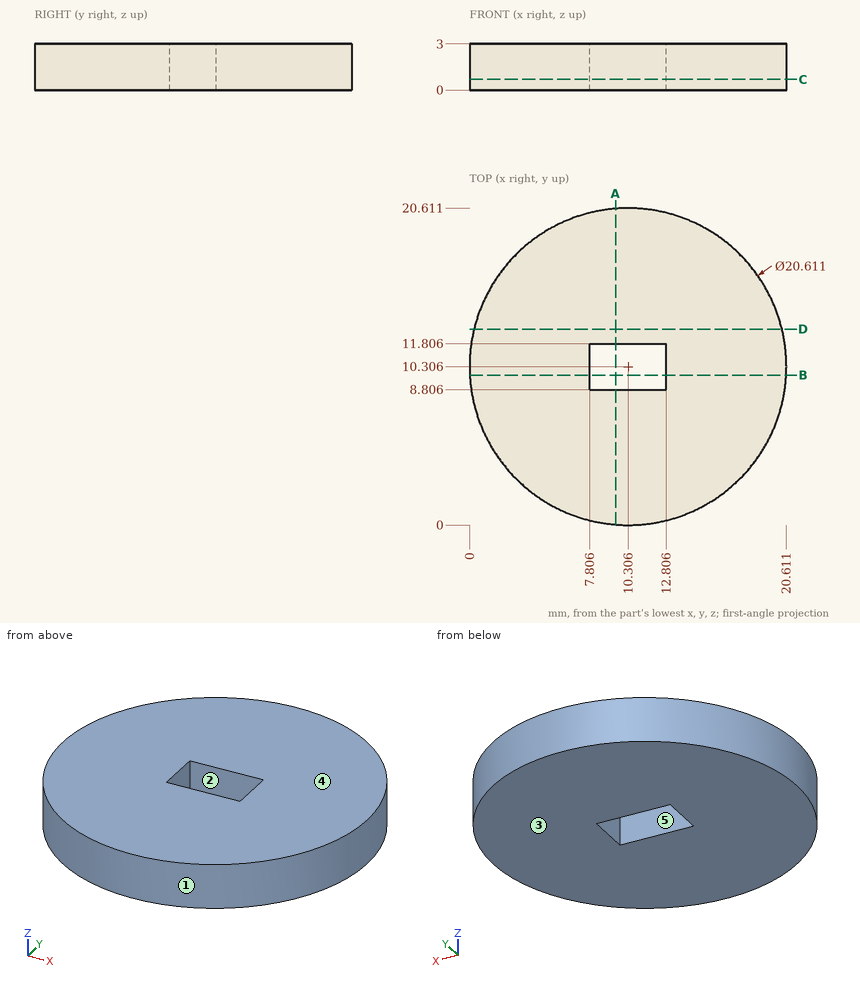
Answer from the drawing. Dimensions are ordinates in mm from the lowest x, y and z of the part. A direction names the side the tool comes from. Round coordinates to 2 decimals unless told otherwise and drop trailing zeros. Write each loop counter-clockwise with the first axis right and the second up, starting at its lowest first coordinate (ties: lowest second). Pieces come first, ordered by that corner, then holes. Notation, with made-up numbers: (73, -25) -> (87, -25) arc R18 ccw to (87, -16) -> close; hole circle Ø10 at (10.5, -6). An arc over 180 degrees is marked (long way). Answer in a Markdown table with one row per item. Add a question column.
1) Which of the six approach directions +Z, -Z, +X, -X, +Y, -Y give full straight-line access (tool end or side, diameter ignored) to the marked faces 4 and 5?
2) Determine the mould class of the marked faces 1, 2 and 3 for opening direction X: pulls with the +X half, pulls with the -X half, needs draft (parallel to the pull), parting line crosses it, or undercut.
3) Find section A-A, the plane x = 9.5. Determine the outline of the cut face in (y, z) (1 decimal).
4) Find section B-B, the plane y = 9.75. Determine the outline of the cut face in (x, z) (1 decimal).
5) Consider line 1 (Y direction, x = 10.25, z = 0.5) (1 decimal); line 2 (Y direction, x = 11.5, z = 2.6) (1 decimal); line 3 (X direction, y = 10.5, z = 0.2) (1 decimal). Determine where each line is inside the solid, lowest interval first.
6) Find section D-D, the plane y = 12.75. Determine the outline of the cut face in (x, z) (1 decimal).
7) Find section C-C, the plane z = 0.7. Determine the outline of the cut face in (x, y) (1 decimal).
8) Given P1, Ø1.5, axis at y = 18, z = 1.5, coming from the +X side; P2, Ø0.9, axis at x = 9.5, z = 1.5, coming from the -Y side; P3, Ø3, axis at x = 5.5, y = 9, coming from the -Z side; P4, Ø1, axis at x = 13, z = 0.5, coming from the +Y side (1 decimal), each flat-ended and moving along its own axis, determine where each tip first touches the part or whether it passes through.
Findings below:
| question | item | result |
|---|---|---|
| 1 | face 4 | +Z, +X, -X, +Y, -Y |
| 1 | face 5 | +Z, -Z |
| 2 | face 1 | parting line crosses it |
| 2 | face 2 | undercut |
| 2 | face 3 | needs draft |
| 3 | outline | (0, 0) -> (8.8, 0) -> (8.8, 3) -> (0, 3) -> close; (11.8, 0) -> (20.6, 0) -> (20.6, 3) -> (11.8, 3) -> close |
| 4 | outline | (0, 0) -> (7.8, 0) -> (7.8, 3) -> (0, 3) -> close; (12.8, 0) -> (20.6, 0) -> (20.6, 3) -> (12.8, 3) -> close |
| 5 | line 1 | 0 to 8.8, 11.8 to 20.6 |
| 5 | line 2 | 0.1 to 8.8, 11.8 to 20.5 |
| 5 | line 3 | 0 to 7.8, 12.8 to 20.6 |
| 6 | outline | (0.3, 0) -> (20.3, 0) -> (20.3, 3) -> (0.3, 3) -> close |
| 7 | outline | circle Ø20.6 at (10.3, 10.3); hole (7.8, 8.8) -> (12.8, 8.8) -> (12.8, 11.8) -> (7.8, 11.8) -> close |
| 8 | P1 | x = 17.92 |
| 8 | P2 | y = 0.01 |
| 8 | P3 | z = 0 |
| 8 | P4 | y = 20.4 |
